Can you work these out from the model? Positions are in its coordinate system, mm. A direction names the side the tool comes from. Give positions to 0.01 mm unless a question says otherwise; leave off trailing zeros. Order: outer loops, then holes, each group sorted by start corner. A loop starts at its lowest first (then second) coordinate and runs counter-clockwise, first axis right, second up. Notation, with made-up numbers: M -30,58.5 L -21,58.5 A22 cw -21,65.5 Z; hole C 54.5,-1 d1. An arc over 180 degrees is marked long. Answer as a JSON object with one key per item and string values.
```python
from build123d import *

# Parameters (mm, degrees)
SKETCH1_W           = 15.24
SKETCH1_H           = 18.796
SKETCH1_R           = 1.27
BOSS_EXTRUDE1_DEPTH = 1.524
SKETCH2_W           = 7.62
SKETCH2_H           = 2.54
BOSS_EXTRUDE2_DEPTH = 2.54
SKETCH4_W           = 0.635
SKETCH4_H           = 0.635
LPATTERN1_COUNT     = 2
LPATTERN1_PITCH     = 2.54
LPATTERN1_COL_COUNT = 2
LPATTERN1_COL_PITCH = 2.54


with BuildPart() as part:
    # Sketch1 → Boss-Extrude1 (new body)
    with BuildSketch(Plane(origin=(0, 0, 0), x_dir=(1, 0, 0), z_dir=(0, 1, 0))):
        Rectangle(SKETCH1_W, SKETCH1_H)
        with Locations((-5.08, 7.239)):
            Circle(SKETCH1_R, mode=Mode.SUBTRACT)
        with Locations((5.08, 7.239)):
            Circle(SKETCH1_R, mode=Mode.SUBTRACT)
    extrude(amount=BOSS_EXTRUDE1_DEPTH)

    # Sketch2 → Boss-Extrude2 (add)
    with BuildSketch(Plane(origin=(0, 1.524, 0), x_dir=(1, 0, 0), z_dir=(0, 1, 0))):
        with Locations((0, -7.366)):
            Rectangle(SKETCH2_W, SKETCH2_H)
    extrude(amount=BOSS_EXTRUDE2_DEPTH)

    # Sweep1: sweep along a path in Sketch3
    with BuildLine(Plane(origin=(0, 0, 0), x_dir=(0, 0, -1), z_dir=(1, 0, 0))) as sweep1_path:
        Line((-7.366, 4.064), (-7.366, 4.953))
        ThreePointArc((-7.366, 4.953), (-7.589184633, 5.491815367), (-8.128, 5.715))
        Line((-8.128, 5.715), (-14.986, 5.715))
    # Sketch4 → Sweep1 (sweep)
    with BuildSketch(Plane.XY.offset(14.986)):
        with Locations((0, 5.715)):
            Rectangle(SKETCH4_W, SKETCH4_H)
    sweep1 = sweep(path=sweep1_path.line)

    # LPattern1: Sweep1 ×2
    with Locations(*[(i * LPATTERN1_PITCH, 0, 0) for i in range(1, LPATTERN1_COUNT)]):
        add(sweep1)

    # LPattern1 col: Sweep1 ×2
    with Locations(*[(-i * LPATTERN1_COL_PITCH, 0, 0) for i in range(1, LPATTERN1_COL_COUNT)]):
        add(sweep1)


solid = part.part
```
1) For faces 1 (the face through (2.858, 5.7, 10.2)), 2 (the face through (-2.858, 5.7, 10.1)), 3 (the face through (0, 3, 6.096)), 4 (the face through (-0.318, 5.7, 10.1)), which set-ups out of +Z, -Z, +X, -X, +Y, -Y let a thin tool reach every point of the face, with its end or its side?
Results found:
{"face 1": "+Z, -Z, +X, +Y", "face 2": "+Z, -Z, -X, +Y", "face 3": "-Z, +X, -X, +Y", "face 4": "+Z, -Z, +Y"}
2) I want a section at D-D on z = 2.5. Write out the boundary of the cut face in (x, y), and give its area (3 significant figures).
Results found:
{"outline": "M -7.62,0 L 7.62,0 L 7.62,1.52 L -7.62,1.52 Z", "area": "23.2 mm²"}
3) I want a section at C-C on x = -5.5. Write out the boundary of the cut face in (y, z), and give its area (3 significant figures).
Results found:
{"outline": "M 0,-9.4 L 1.52,-9.4 L 1.52,-8.44 L 0,-8.44 Z; M 0,-6.04 L 1.52,-6.04 L 1.52,9.4 L 0,9.4 Z", "area": "25.0 mm²"}
4) I need wall thicknesses on L1, parallel to X at y = 5.5, z = 7.75; L2, parallel to Z at x = 5.08, y = 1.1; L3, parallel to Z at x = -1.75, y = 2. Which ranges of each line are inside material? Lowest first, please.
Results found:
{"L1": "x = -2.86 to -2.22, -0.32 to 0.32, 2.22 to 2.86", "L2": "z = -9.4 to -8.51, -5.97 to 9.4", "L3": "z = 6.1 to 8.64"}
5) I want a section at A-A on x = 5.08. Write out the boundary of the cut face in (y, z).
Results found:
{"outline": "M 0,-9.4 L 1.52,-9.4 L 1.52,-8.51 L 0,-8.51 Z; M 0,-5.97 L 1.52,-5.97 L 1.52,9.4 L 0,9.4 Z"}
6) I want a section at B-B on z = 10.75. Write out the boundary of the cut face in (x, y).
Results found:
{"outline": "M -2.86,5.4 L -2.22,5.4 L -2.22,6.03 L -2.86,6.03 Z; M -0.32,5.4 L 0.32,5.4 L 0.32,6.03 L -0.32,6.03 Z; M 2.22,5.4 L 2.86,5.4 L 2.86,6.03 L 2.22,6.03 Z"}
7) I'm going to push flat-ended pins straight in: pin 1 Ø7.5 at (x, z) = (-2, 0.5) entering from +Y; pin 2 Ø1 at (y, z) = (5, 9) entering from -X; pin 3 Ø0.6 at (y, z) = (5.5, 12.5) entering from +X. Where does each tip first touch, or does it pass through?
Results found:
{"pin 1": "stops at y = 1.52", "pin 2": "stops at x = -2.86", "pin 3": "stops at x = 2.86"}
